```python
from build123d import *

# Parameters (mm, degrees)
F2_DEPTH = 6.35


# Not quite as in the source:
# - a feature of the source that left no trace in its solid (it failed there, or was rolled back) is left out
# - a feature names something its author has since deleted; it is built from what else it names


with BuildPart() as f2:
    # F0 (on Front) → F2 (new body)
    with BuildSketch(Plane.XZ):
        with BuildLine():
            Line((6.35, -22.225), (22.225, -22.225))
            Line((22.225, -22.225), (22.225, 22.225))
            Line((22.225, 22.225), (0, 22.225))
            ThreePointArc((0, 22.225), (-15.7154482119, 15.7154482119), (-22.225, 0))
            ThreePointArc((-22.225, 0), (-17.8196433045, -13.2819779212), (-6.35, -21.2985474857))
            Line((-6.35, -21.2985474857), (-6.35, 0))
            ThreePointArc((-6.35, 0), (0, 6.35), (6.35, 0))
            Line((6.35, 0), (6.35, -22.225))
        make_face()
    extrude(amount=F2_DEPTH)


with BuildPart() as f2_1:
    # F3: moved
    add(f2.part.moved(Location((-22.225, -50.8, 0))))


solid = f2_1.part
```
The listing builds one solid part. Answer for the finished solid, in the listing's coordinates (mm). A direction names the side the tool comes from. Coordinates: 2 decimals unless noted, no trailing zeros. Order: outer loops, then holes, each group sorted by start corner. A loop starts at its lowest first (then second) coordinate and runs counter-clockwise, first axis right, second up. Notation, with made-up numbers: M -23,40.25 L -15,40.25 A30 cw -15,66.25 Z; hole C -29.5,-15.75 d5. An arc over 180 degrees is marked long. Answer as a JSON object with one key per item and string values. Group by question number.
1. Section C-C on z = -18 is taken. Write down the section's boundary in (x, y) (3 decimals), then the cut area to 3 significant figures.
2. Determine the mould class of faces 1 (the cylindrical face through (-22.36, -53.93, 6.35)), 2 (the cylindrical face through (-44.15, -53.93, 3.65)), 3 (the flat face through (-11, -54, 22.225)) for opening direction X: released by +X, released by -X, zero draft, split by the parting line, or undercut.
3. Section A-A on z = -6.5 is taken. Write down the section's boundary in (x, y) (3 decimals).
4. Section D-D on x = -41 is taken. Write down the section's boundary in (y, z).
5. Straight lines are drawn through the part: line 1 (X direction, y = -53.5, z = -20) (3 decimals); line 2 (X direction, y = -55.75, z = -14.5) (3 decimals); line 3 (Z direction, x = -17, y = -51.25) (3 decimals). For each, find the intervals that lie inside material, in ascending order.
6. Section B-B on y = -56.25 is taken. Write down the section's boundary in (x, z) (3 decimals).
7. A tool of negligible diameter and unlimited length cuts with its end or side. For faces 4 (the flat face through (-18, -57.15, 5)), 5 (the flat face through (-28.575, -54, -11)), from which of +Z, -Z, +X, -X, +Y, -Y can it reach the whole face along a straight path? Write none if from no direction.
8. Flat-ended cylindrical pins translate along their axes: P1, Ø3, axis at x = -38, y = -54.5, coming from the -Z side; P2, Ø1.9, axis at y = -54, z = -9, coming from the -X side; P3, Ø1, axis at x = -31.5, y = -55, coming from the -Z side. Find the tip coordinate at first contact, or state that the pin passes through.
Values follow:
{
 "1": {"outline": "M -35.262,-57.15 L -28.575,-57.15 L -28.575,-50.8 L -35.262,-50.8 Z; M -15.875,-57.15 L 0,-57.15 L 0,-50.8 L -15.875,-50.8 Z", "area": "143 mm2"},
 "2": {"face 1": "undercut", "face 2": "released by -X", "face 3": "zero draft"},
 "3": {"outline": "M -43.478,-57.15 L -28.575,-57.15 L -28.575,-50.8 L -43.478,-50.8 Z; M -15.875,-57.15 L 0,-57.15 L 0,-50.8 L -15.875,-50.8 Z"},
 "4": {"outline": "M -57.15,-11.89 L -50.8,-11.89 L -50.8,11.89 L -57.15,11.89 Z"},
 "5": {"line 1": "-31.918 to -28.575, -15.875 to 0", "line 2": "-39.068 to -28.575, -15.875 to 0", "line 3": "3.609 to 22.225"},
 "6": {"outline": "M -28.575,-21.299 L -28.575,0 A6.35 cw -15.875,0 L -15.875,-22.225 L 0,-22.225 L 0,22.225 L -22.225,22.225 A22.225 ccw Z"},
 "7": {"face 4": "+Z, -Z, +X, -X, -Y", "face 5": "-Z, +Y, -Y"},
 "8": {"P1": "z = -17.03", "P2": "x = -42.94", "P3": "z = -20.42"}
}
